from build123d import *

# Parameters (mm, degrees)
BOX001_W          = 10
BOX001_H          = 100
BOX001_DEPTH      = 5
CYLINDER004_R     = 1.5
CYLINDER004_DEPTH = 10
CYLINDER005_R     = 1.5
CYLINDER005_DEPTH = 10
CYLINDER006_R     = 1.5
CYLINDER006_DEPTH = 10
CYLINDER007_R     = 5
CYLINDER007_DEPTH = 5
CYLINDER002_R     = 4.5
CYLINDER002_DEPTH = 5
CYLINDER003_R     = 4.5
CYLINDER003_DEPTH = 5
BOX_W             = 35
BOX_H             = 30.5
BOX_DEPTH         = 5
CYLINDER_R        = 8.5
CYLINDER_DEPTH    = 5
CYLINDER001_R     = 17.5
CYLINDER001_DEPTH = 5


with BuildPart() as cube001:
    # Box001 → Box001 (new body)
    with BuildSketch(Plane(origin=(-5, -113, 0), x_dir=(1, 0, 0), z_dir=(0, 0, 1))):
        with Locations((5, 50)):
            Rectangle(BOX001_W, BOX001_H)
    extrude(amount=BOX001_DEPTH)


with BuildPart() as cylinder004:
    # Cylinder004 → Cylinder004 (new body)
    with BuildSketch(Plane(origin=(0, -13, 5), x_dir=(1, 0, 0), z_dir=(0, 0, 1))):
        Circle(CYLINDER004_R)
    extrude(amount=CYLINDER004_DEPTH)


with BuildPart() as cylinder005:
    # Cylinder005 → Cylinder005 (new body)
    with BuildSketch(Plane(origin=(13, 0, 5), x_dir=(1, 0, 0), z_dir=(0, 0, 1))):
        Circle(CYLINDER005_R)
    extrude(amount=CYLINDER005_DEPTH)


with BuildPart() as cylinder006:
    # Cylinder006 → Cylinder006 (new body)
    with BuildSketch(Plane(origin=(-13, 0, 5), x_dir=(1, 0, 0), z_dir=(0, 0, 1))):
        Circle(CYLINDER006_R)
    extrude(amount=CYLINDER006_DEPTH)


with BuildPart() as cylinder007:
    # Cylinder007 → Cylinder007 (new body)
    with BuildSketch(Plane(origin=(0, -113, 0), x_dir=(1, 0, 0), z_dir=(0, 0, 1))):
        Circle(CYLINDER007_R)
    extrude(amount=CYLINDER007_DEPTH)


with BuildPart() as cylinder002:
    # Cylinder002 → Cylinder002 (new body)
    with BuildSketch(Plane(origin=(13, 0, 0), x_dir=(1, 0, 0), z_dir=(0, 0, 1))):
        Circle(CYLINDER002_R)
    extrude(amount=CYLINDER002_DEPTH)


with BuildPart() as cylinder003:
    # Cylinder003 → Cylinder003 (new body)
    with BuildSketch(Plane(origin=(-13, 0, 0), x_dir=(1, 0, 0), z_dir=(0, 0, 1))):
        Circle(CYLINDER003_R)
    extrude(amount=CYLINDER003_DEPTH)


with BuildPart() as cube:
    # Box → Box (new body)
    with BuildSketch(Plane(origin=(-17.5, 0, 0), x_dir=(1, 0, 0), z_dir=(0, 0, 1))):
        with Locations((17.5, 15.25)):
            Rectangle(BOX_W, BOX_H)
    extrude(amount=BOX_DEPTH)


with BuildPart() as cylinder:
    # Cylinder → Cylinder (new body)
    with BuildSketch(Plane.XY):
        Circle(CYLINDER_R)
    extrude(amount=CYLINDER_DEPTH)


with BuildPart() as obj1:
    # Cylinder001 → Cylinder001 (new body)
    with BuildSketch(Plane.XY):
        Circle(CYLINDER001_R)
    extrude(amount=CYLINDER001_DEPTH)

    # Cut: cut Cylinder
    add(cylinder.part, mode=Mode.SUBTRACT)

    # Cut001: cut Cube
    add(cube.part, mode=Mode.SUBTRACT)

    # Fusion: union Cylinder002, Cylinder003
    add(cylinder002.part)
    add(cylinder003.part)

    # Fusion001: union Cube001, Cylinder004, Cylinder005, Cylinder006, Cylinder007
    add(cube001.part)
    add(cylinder004.part)
    add(cylinder005.part)
    add(cylinder006.part)
    add(cylinder007.part)


solid = obj1.part
Geometry check sheet. Reference: the model listing, model coordinates, mm. A direction names the side the tool comes from. Coordinates: 2 decimals unless noted, no trailing zeros. Loops run counter-clockwise (first coordinate to the right, second up) from the corner with the lowest first, then second, coordinate; pieces in that order, holes last. Notation, with made-up numbers: (73.5, -19) - (98.5, -19) arc R17 cw to (98.5, -6) - close; hole circle Ø8 at (38.5, 49.5). An arc over 180 degrees is marked (long way). Use one line per item in the form item = value. Start each with the question number.
Item 1: Gauge pin test, flat ends, axial feed: pin 1 (6 mm diameter, centred on y = -64, z = 5.5, fed in from -X); pin 2 (12 mm diameter, centred on x = 6.5, y = -83, fed in from +Z); pin 3 (6 mm diameter, centred on y = -43.5, z = 4, fed in from +X). Record the tip position at first contact, or that the pin passes through.
Item 2: Thickness scan on probe 1 along Z at (x, y) = (-4.5, -8); probe 2 along X at (y, z) = (-82, 1.5); probe 3 along Y at (x, z) = (-11.5, 3.75). Record the ranges inside material, lowest first.
Item 3: Mould release check, pull along X, two halves, no side actions. Record for faces 4 (the face through (13.1, 4.5, 2.5)), 5 (the face through (13.94, -10.58, 2.46)), 6 (the face through (0, -118, 2)), 7 (the face through (0, -13, 15)): +X half, -X half, draft (parallel to the pull), parting line (faces both ways), or undercut.
Item 4: Section check C-C, the plane y = -13. Enter the section's corners in (x, z), and give its area (3 significant figures).
Item 5: Section check D-D, the plane y = -44.5. Enter the section's corners in (x, z), and give its area (3 significant figures).
Item 6: Tool access check on faces 1 (the face through (-5, -66, 2)), 2 (the face through (-0.325, -14.464, 9.93)), 3 (the face through (5, -66, 2)). Record the directions out of +Z, -Z, +X, -X, +Y, -Y that give a thin tool (end or side, any length) a straight path to the whole face; none if there is none.
Item 7: Section check A-A, the plane x = 0. Enter the section's corners in (y, z), and give its area (4 significant figures).
Item 8: Section check B-B, the plane z = 10. Enter the section's corners in (x, y).
Computed:
q1.pin_1 = -5
q1.pin_2 = 5
q1.pin_3 = 5
q2.probe_1 = 0 to 5
q2.probe_2 = -5 to 5
q2.probe_3 = -13.19 to 4.24
q3.face_4 = undercut
q3.face_5 = +X half
q3.face_6 = parting line
q3.face_7 = draft
q4.outline = (-11.72, 0) - (11.72, 0) - (11.72, 5) - (1.5, 5) - (1.5, 15) - (-1.5, 15) - (-1.5, 5) - (-11.72, 5) - close
q4.area = 147 mm2
q5.outline = (-5, 0) - (5, 0) - (5, 5) - (-5, 5) - close
q5.area = 50.0 mm2
q6.face_1 = +Z, -Z, -X, -Y
q6.face_2 = +Z
q6.face_3 = +Z, -Z, +X, -Y
q7.outline = (-118, 0) - (-8.5, 0) - (-8.5, 5) - (-11.5, 5) - (-11.5, 15) - (-14.5, 15) - (-14.5, 5) - (-118, 5) - close
q7.area = 577.5 mm2
q8.outline = circle Ø3 at (-13, 0); circle Ø3 at (0, -13); circle Ø3 at (13, 0)
